Autodesk Inventor part; units mm, degrees
ref_plane "YZ Plane" through (0, 0, 0) normal (1, 0, 0) x (0, 1, 0)
ref_plane "XZ Plane" through (0, 0, 0) normal (0, 1, 0) x (-1, 0, 0)
ref_plane "XY Plane" through (0, 0, 0) normal (0, 0, 1) x (1, 0, 0)
sketch "Sketch1" plane through (0, 0, 0) normal (0, 0, 1) x (1, 0, 0)
  line L0 (-106.5, -15.5) -> (106.5, -15.5)
  line L1 (106.5, -15.5) -> (106.5, 15.5)
  line L2 (106.5, 15.5) -> (-106.5, 15.5)
  line L3 (-106.5, 15.5) -> (-106.5, -15.5)
  line L4 (-106.5, -15.5) -> (106.5, 15.5) construction
  line L5 (106.5, -15.5) -> (-106.5, 15.5) construction
  point P0 (0, 0)
  dimension "L" = 213
  dimension "d1" = 31
extrude "Extrusion1" add sketch "Sketch1" along normal blind 20
sketch "Sketch2" plane through (106.5, -15.5, 0) normal (1, 0, 0) x (0, 0, -1)
  line L0 (0, 0) -> (-20, 0)
  line L1 (0, 0) -> (-20, 15.5)
  line L2 (-20, 0) -> (-20, 31)
  point P0 (0, 15.5)
extrude "Extrusion2" cut sketch "Sketch2" against normal through all
mirror "Mirror1" about plane through (0, 0, 0) normal (0, 1, 0) of "Extrusion2"
sketch "Sketch3" plane through (0, 0, 0) normal (0, 1, 0) x (-1, 0, 0)
  line L0 (106.5, 0) -> (-106.5, 0)
  line L1 (-106.5, 0) -> (-96.5, 20)
  line L2 (106.5, 20) -> (-106.5, 20)
  line L3 (-106.5, 0) -> (-106.5, 20)
  point P0 (0, 0)
  dimension "d6" = 10
extrude "Extrusion3" cut sketch "Sketch3" along normal through all both and the other way through all
mirror "Mirror2" about plane through (0, 0, 0) normal (1, 0, 0) of "Extrusion3"
shell "Shell1" thickness 2.5 removed faces 2 at (-32.1667, -10.3333, 6.6667) at (35.5, -5.1667, 0)
sketch "Sketch4" plane through (0, 0, 0) normal (0, 0, 1) x (1, 0, 0)
  line L0 (-106.5, -15.5) -> (-103.7049, -15.5)
  line L1 (-103.7049, -15.5) -> (-85.5, 12.3371)
  line L2 (103.7049, 12.3371) -> (-103.7049, 12.3371)
  line L3 (-106.5, 15.5) -> (-106.5, -15.5)
  line L4 (-103.7049, 12.3371) -> (-103.7049, -15.5)
  point P0 (0, 0)
  dimension "d10" = 21
extrude "Extrusion4" add sketch "Sketch4" along normal up to surface surface through (106.5, -1.976, 18.4686) normal (0, -0.7904151, -0.6125717)
ref_plane "Work Plane1" through (-106.5, -15.5, 0) normal (-0.8944272, 0, 0.4472136) x (0.4472136, 0, 0.8944272)
split "Split1" plane through (-106.5, -15.5, 0) removes the side toward (-0.8944272, 0, 0.4472136)
ref_plane "Work Plane2" through (-96.5, 0, 20) normal (0, -0.7904151, 0.6125717) x (1, 0, 0)
split "Split2" plane through (-96.5, 0, 20) removes the side toward (0, -0.7904151, 0.6125717)
mirror "Mirror3" about plane through (0, 0, 0) normal (1, 0, 0) of "Extrusion4", "Split1", "Split2"
fillet "Fillet1" radius 0.3 4 edges at (-101.5, 7.75, 10) (-101.5, -7.75, 10) (101.5, 7.75, 10) (101.5, -7.75, 10)
fillet "Fillet2" radius 0.3 3 edges at (96.4817, 0, 19.9011) (-96.4817, 0, 19.9011) (0, 0, 20)
sketch "Sketch5" plane through (0, 0, 0) normal (0, 0, -1) x (-1, 0, 0)
  line L0 (-96, 3.5) -> (96, 3.5)
  line L1 (-106.2565, 15.5) -> (106.2565, 15.5)
  point P0 (0, 0)
  point P1 (0, 3.5)
  dimension "d17" = 12
  dimension "BC" = 192
hole "Hole1" at (96, 3.5, 0) at (-96, 3.5, 0) direction (0, 0, 1) diameter 3.242 depth 11 tip angle 118
chamfer "Chamfer1" distance 0.2 angle 45 2 edges at (96, 1.879, 0) (-96, 1.879, 0)
ref_plane "Work Plane3" through (106.5, -15.5, 0) normal (-0.8944272, 0, -0.4472136) x (-0.4472136, 0, 0.8944272)
properties part number "ESTAMP Post 6832 Gold L=149; BC=128" material "Zinc"
Here's how the part is built. I have some questions about the finished solid (model axes, mm). A direction names the side the tool comes from. Round coordinates to 2 decimals unless told otherwise and drop trailing zeros. Write each loop counter-clockwise with the first axis right and the second up, starting at its lowest first coordinate (ties: lowest second). Pieces come first, ordered by that corner, then holes.
1. Suppose I cut it at B-B (z = 9.25). State how many separate pieces and enclosed holes the cut face has, and give its area (3 significant figures).
2. I need wall thicknesses on L1, parallel to X at y = 3.5, z = 6.75 (3 decimals); L2, parallel to X at y = 4.5, z = 3.75 (3 decimals); L3, parallel to Y at x = 96, z = 3.25. Which ranges of each line are inside material? Lowest first, please.
3. Will these pins go through, and if not, where does the flat tip stop? pin 1 Ø2 at (x, z) = (-79, 11) entering from -Y; pin 2 Ø3.5 at (x, y) = (-96, 3.5) entering from +Z; pin 3 Ø2 at (x, z) = (38.5, 12) entering from +Y (3 decimals); pin 4 Ø8 at (x, y) = (-84.5, 4) entering from +Z.
4. For faces 1 (the flat face through (94.475, -1.387, 6.859)), 2 (the flat face through (0, 14, 0)), which set-ups out of +Z, -Z, +X, -X, +Y, -Y let a thin tool reach every point of the face, with its end or its side?
5. Suppose I cut it at A-A (x = -26.5). List the corners of the cut face in (y, z) for me.
Answer sheet:
1. separate pieces: 1
1. enclosed holes: 2
1. area: 824 mm2
2. L1: x = -103.125 to -97.621, -94.379 to -91.279, 91.279 to 94.379, 97.621 to 103.125
2. L2: x = -104.625 to -97.276, -94.724 to -90.625, 90.625 to 94.724, 97.276 to 104.625
2. L3: y = -3.72 to 1.88, 5.12 to 12.98
3. pin 1: stops at y = 3.04
3. pin 2: stops at z = 17.74
3. pin 3: stops at y = 6.975
3. pin 4: stops at z = 19.81
4. face 1: -Z, -Y
4. face 2: -Z, +X, -X, +Y, -Y
5. outline: (-1.58, 17.96) - (12.34, 0) - (15.5, 0) - (0.24, 19.69) arc R0.3 ccw to (-0.24, 19.69) - close
